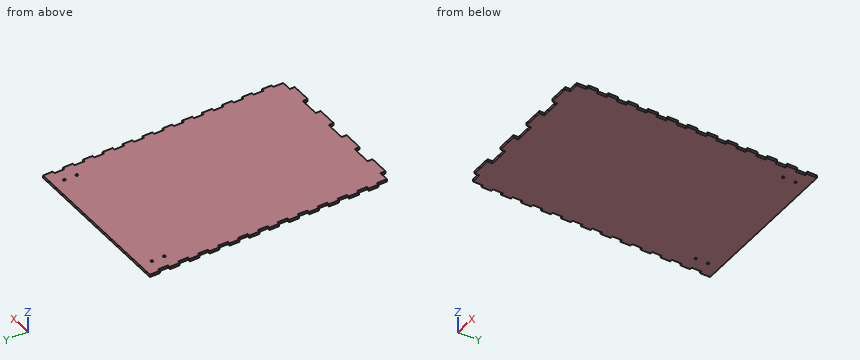
```python
from build123d import *

# Parameters (mm, degrees)
SKETCH1_W           = 203.2
SKETCH1_H           = 304.8
BOSS_EXTRUDE1_DEPTH = 3.175
SKETCH2_W           = 3.175
SKETCH2_H           = 12.7
SKETCH2_W_2         = 25.4
SKETCH2_H_2         = 6.35
BOSS_EXTRUDE2_DEPTH = 3.175
SKETCH5_R           = 1.5
CUT_EXTRUDE2_DEPTH  = 3.175


with BuildPart() as part:
    # Sketch1 → Boss-Extrude1 (new body)
    with BuildSketch(Plane.XY):
        with Locations((101.6, 152.4)):
            Rectangle(SKETCH1_W, SKETCH1_H)
    extrude(amount=BOSS_EXTRUDE1_DEPTH)

    # Sketch2 → Boss-Extrude2 (add)
    with BuildSketch(Plane.XY.offset(3.175)):
        with Locations((-1.5875, 298.45)):
            Rectangle(SKETCH2_W, SKETCH2_H)
        with Locations((204.7875, 298.45)):
            Rectangle(SKETCH2_W, SKETCH2_H)
        with Locations((-1.5875, 273.05)):
            Rectangle(SKETCH2_W, SKETCH2_H)
        with Locations((204.7875, 273.05)):
            Rectangle(SKETCH2_W, SKETCH2_H)
        with Locations((-1.5875, 247.65)):
            Rectangle(SKETCH2_W, SKETCH2_H)
        with Locations((204.7875, 247.65)):
            Rectangle(SKETCH2_W, SKETCH2_H)
        with Locations((-1.5875, 222.25)):
            Rectangle(SKETCH2_W, SKETCH2_H)
        with Locations((204.7875, 222.25)):
            Rectangle(SKETCH2_W, SKETCH2_H)
        with Locations((-1.5875, 196.85)):
            Rectangle(SKETCH2_W, SKETCH2_H)
        with Locations((204.7875, 196.85)):
            Rectangle(SKETCH2_W, SKETCH2_H)
        with Locations((-1.5875, 171.45)):
            Rectangle(SKETCH2_W, SKETCH2_H)
        with Locations((204.7875, 171.45)):
            Rectangle(SKETCH2_W, SKETCH2_H)
        with Locations((-1.5875, 146.05)):
            Rectangle(SKETCH2_W, SKETCH2_H)
        with Locations((204.7875, 146.05)):
            Rectangle(SKETCH2_W, SKETCH2_H)
        with Locations((-1.5875, 120.65)):
            Rectangle(SKETCH2_W, SKETCH2_H)
        with Locations((204.7875, 120.65)):
            Rectangle(SKETCH2_W, SKETCH2_H)
        with Locations((-1.5875, 95.25)):
            Rectangle(SKETCH2_W, SKETCH2_H)
        with Locations((204.7875, 95.25)):
            Rectangle(SKETCH2_W, SKETCH2_H)
        with Locations((-1.5875, 69.85)):
            Rectangle(SKETCH2_W, SKETCH2_H)
        with Locations((204.7875, 69.85)):
            Rectangle(SKETCH2_W, SKETCH2_H)
        with Locations((-1.5875, 44.45)):
            Rectangle(SKETCH2_W, SKETCH2_H)
        with Locations((204.7875, 44.45)):
            Rectangle(SKETCH2_W, SKETCH2_H)
        with Locations((-1.5875, 19.05)):
            Rectangle(SKETCH2_W, SKETCH2_H)
        with Locations((204.7875, 19.05)):
            Rectangle(SKETCH2_W, SKETCH2_H)
        with Locations((25.4, -3.175)):
            Rectangle(SKETCH2_W_2, SKETCH2_H_2)
        with Locations((76.2, -3.175)):
            Rectangle(SKETCH2_W_2, SKETCH2_H_2)
        with Locations((127, -3.175)):
            Rectangle(SKETCH2_W_2, SKETCH2_H_2)
        with Locations((177.8, -3.175)):
            Rectangle(SKETCH2_W_2, SKETCH2_H_2)
    extrude(amount=-BOSS_EXTRUDE2_DEPTH)

    # Sketch5 → Cut-Extrude2 (cut)
    with BuildSketch(Plane(origin=(0, 0, 0), x_dir=(-1, 0, 0), z_dir=(0, 0, -1))):
        with Locations((-187.325, 289.8)):
            Circle(SKETCH5_R)
        with Locations((-187.325, 274.05)):
            Circle(SKETCH5_R)
        with Locations(Location((-15.875, 274.05, 0), (0, 0, 180))):
            Circle(SKETCH5_R)
        with Locations(Location((-15.875, 289.8, 0), (0, 0, 180))):
            Circle(SKETCH5_R)
    extrude(amount=-CUT_EXTRUDE2_DEPTH, mode=Mode.SUBTRACT)


solid = part.part
```
For this review, take the finished solid that the model builds, in its own axes (mm). Coordinates: 2 decimals unless noted, no trailing zeros. Order: outer loops, then holes, each group sorted by start corner. A loop starts at its lowest first (then second) coordinate and runs counter-clockwise, first axis right, second up. Notation, with made-up numbers: (-38, -37.75) - (8, -37.75) arc R20 ccw to (8, -32.75) - close; hole circle Ø8 at (-17, 41.25). An arc over 180 degrees is marked (long way). Answer as a JSON object with one key per item and string values. Group by question number.
1. Clearance check with flat-ended pins moving along their axes: P1, Ø1.6, axis at y = 85, z = 1, coming from the -X side; P2, Ø1.6, axis at y = -3, z = 1, coming from the +X side; P3, Ø1, axis at y = 262.5, z = 1, coming from the +X side. State where each tip first meets the part, or that it passes through.
2. We need section A-A on z = 1.9. Give the number of separate pieces and of enclosed holes in the cut face, then the cut area to 3 significant figures.
3. For probe 1 along X at (y, z) = (274.05, 2.5) (3 decimals); probe 2 along X at (y, z) = (289.8, 2.55) (3 decimals); probe 3 along Y at (x, z) = (96, 0.2), list the stretches that pass through material, from the lowest coordinate up.
4. We need section B-B on x = 98. State the section outline as (y, z) points (3 decimals), then the cut area to 3 significant figures.
Final values:
{
 "1": {"P1": "x = 0", "P2": "x = 190.5", "P3": "x = 203.2"},
 "2": {"separate pieces": "1", "enclosed holes": "4", "area": "63,500 mm²"},
 "3": {"probe 1": "-3.175 to 14.375, 17.375 to 185.825, 188.825 to 206.375", "probe 2": "0 to 14.375, 17.375 to 185.825, 188.825 to 203.2", "probe 3": "0 to 304.8"},
 "4": {"outline": "(0, 0) - (304.8, 0) - (304.8, 3.175) - (0, 3.175) - close", "area": "968 mm²"}
}
